from build123d import *

# Parameters (mm, degrees)
EXTRUDE_1_DEPTH     = 754
CUT_EXTRUDE_1_DEPTH = 60


with BuildPart() as part:
    # Эскиз1 → Вытянуть-Тонкостенный1 (new body)
    with BuildSketch(Plane.XY):
        with BuildLine():
            Line((-40, 39), (-40, -39))
            ThreePointArc((-40, -39), (-38.242640687, -43.242640687), (-34, -45))
            Line((-34, -45), (34, -45))
            ThreePointArc((34, -45), (38.242640687, -43.242640687), (40, -39))
            Line((40, -39), (40, 39))
            ThreePointArc((40, 39), (38.242640687, 43.242640687), (34, 45))
            Line((34, 45), (-34, 45))
            ThreePointArc((-34, 45), (-38.242640687, 43.242640687), (-40, 39))
        make_face()
        with BuildLine():
            Line((-37, 39), (-37, -39))
            ThreePointArc((-37, -39), (-36.121320344, -41.121320344), (-34, -42))
            Line((-34, -42), (34, -42))
            ThreePointArc((34, -42), (36.121320344, -41.121320344), (37, -39))
            Line((37, -39), (37, 39))
            ThreePointArc((37, 39), (36.121320344, 41.121320344), (34, 42))
            Line((34, 42), (-34, 42))
            ThreePointArc((-34, 42), (-36.121320344, 41.121320344), (-37, 39))
        make_face(mode=Mode.SUBTRACT)
    extrude(amount=EXTRUDE_1_DEPTH)

    # Эскиз2 → Вырез-Вытянуть1 (cut, symmetric)
    with BuildSketch(Plane(origin=(0, 0, 0), x_dir=(1, 0, 0), z_dir=(0, 1, 0))):
        Polygon((40, 0), (-40, -155.555555538), (-177.752070978, 72.913369191), (175.578140708, 72.913369191), (175.578140708, -903.068684068), (-185.164592902, -903.068684068), (-40, -712.857142852), (40, -754), align=None)
    extrude(amount=CUT_EXTRUDE_1_DEPTH, both=True, mode=Mode.SUBTRACT)


solid = part.part
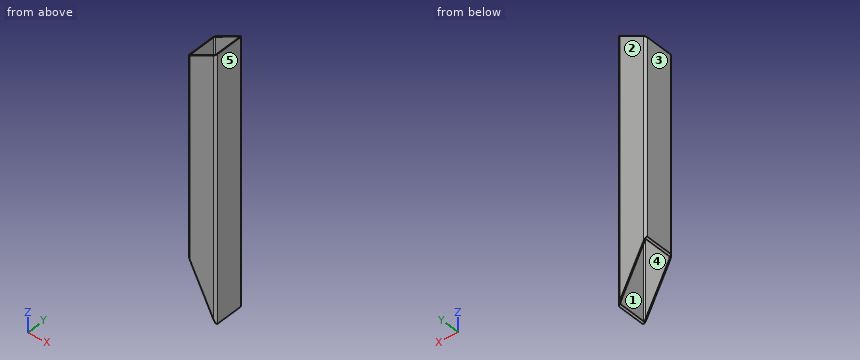
Check sheet for the modelled part. Datum: model origin and axes. Units: mm. Face numbers are marked on the shaded views. A direction names the side the tool comes from. Give positions to 0.01 mm unless a question says otherwise; leave off trailing zeros. Loops run counter-clockwise (first coordinate to the right, second up) from the corner with the lowest first, then second, coordinate; pieces in that order, holes last. Notation, with made-up numbers: M 65.25,68.25 L 70.25,68.25 A18 ccw 70.25,86.25 Z; hole C 24.25,44 d6. An arc over 180 degrees is marked long. Return JSON: item names as keys, results as strings. Group by question number.
1. Cross-section at B-B on z = 269.5. Record the boundary of the cut face in (x, y), plus the area to 3 significant figures.
2. Cross-section at D-D on z = 111. Record the boundary of the cut face in (x, y).
3. Cross-section at C-C on x = -24. Record the boundary of the cut face in (y, z), plus the area to 3 significant figures.
4. Cross-section at A-A on y = 30. Record the boundary of the cut face in (x, z).
5. Thickness scan on L1, parallel to X at y = 17.5, z = 423; L2, parallel to Y at x = -15.5, z = 235; L3, parallel to X at y = -41, z = 178.5. Record the ranges inside material, lowest first.
6. Mould release check, pull along X, two halves, no side actions. Record for the marked faces 3, 4 and 5: released by +X, released by -X, zero draft, split by the parting line, or undercut.
7. Tool access check on the marked faces 1 and 2. Record the directions out of +Z, -Z, +X, -X, +Y, -Y that give a thin tool (end or side, any length) a straight path to the whole face; none if there is none.
Return value:
{
 "1": {"outline": "M -40,-39 A6 ccw -34,-45 L 34,-45 A6 ccw 40,-39 L 40,39 A6 ccw 34,45 L -34,45 A6 ccw -40,39 Z; hole M -37,-39 A3 ccw -34,-42 L 34,-42 A3 ccw 37,-39 L 37,39 A3 ccw 34,42 L -34,42 A3 ccw -37,39 Z", "area": "961 mm^2"},
 "2": {"outline": "M -17.09,-45 L 34,-45 A6 ccw 40,-39 L 40,39 A6 ccw 34,45 L -17.09,45 L -17.09,42 L 34,42 A3 cw 37,39 L 37,-39 A3 cw 34,-42 L -17.09,-42 Z"},
 "3": {"outline": "M -45,124.44 L -42,124.44 L -42,721.09 L -45,721.09 Z; M 42,124.44 L 45,124.44 L 45,721.09 L 42,721.09 Z", "area": "3,580 mm^2"},
 "4": {"outline": "M -40,155.56 L -37,149.72 L -37,714.4 L -40,712.86 Z; M 37,5.83 L 40,0 L 40,754 L 37,752.46 Z"},
 "5": {"L1": "-40 to -37, 37 to 40", "L2": "-45 to -42, 42 to 45", "L3": "-39.66 to -36.24, 36.24 to 39.66"},
 "6": {"face 3": "released by -X", "face 4": "undercut", "face 5": "released by +X"},
 "7": {"face 1": "+Z, -Z", "face 2": "+Z, -Z, +X, -X, +Y"}
}
